Source: CAD feature listing. Evaluate the final solid. Frame: model axes, mm. Coordinates: 2 decimals unless noted, no trailing zeros. Loops run counter-clockwise (first coordinate to the right, second up) from the corner with the lowest first, then second, coordinate; pieces in that order, holes last. Notation, with made-up numbers: (41.5, 49) - (50.5, 49) arc R18 ccw to (50.5, 81) - close; hole circle Ø10 at (-8.75, 81). An arc over 180 degrees is marked (long way). Use CSV: the item, a comma, the result in double quotes. Start each with the question number.
```python
from build123d import *

# Parameters (mm, degrees)
F0_R     = 38.572234299
F1_DEPTH = 25.4
F2_DEPTH = 25.4
F3_DEPTH = 25.4


with BuildPart() as f1:
    # F0 (on Front) → F1 (new body)
    with BuildSketch(Plane.XZ):
        with Locations((-53.8619197905, 27.4006854743)):
            Circle(F0_R)
    extrude(amount=F1_DEPTH)

    # F2 (add): faces of the model
    f2_faces = [f1.faces().sort_by_distance(p)[0] for p in [
        (-53.8619197905, -25.4, 27.4006854743),
        (-53.8619197905, 0, 27.4006854743),
    ]]
    extrude(f2_faces, amount=F2_DEPTH, dir=(0, -1, 0))

    # F3 (add): a face of the model
    f3_faces = [f1.faces().sort_by_distance(p)[0] for p in [
        (-53.8619197905, 0, 27.4006854743),
    ]]
    extrude(f3_faces, amount=F3_DEPTH)


solid = f1.part
```
(1) Pin query (flat end, axial travel): pin 1 Ø3 at (y, z) = (-14.5, 33.5) entering from +X; pin 2 Ø1 at (x, y) = (-49.5, 8) entering from +Z; pin 3 Ø4 at (x, y) = (-38.5, -1) entering from -Z. Return the tip coordinate at first contact, or that it passes through.
(2) Section A-A on x = -22. Output: boundary loops of the cut face in (y, z), plus the area to 3 significant figures.
(3) Ray query, line 1 (Z direction, x = -53.5, y = 18); line 2 (Z direction, x = -34, y = -12.5); line 3 (X direction, y = -10, z = -2). Return the intervals inside material, ascending. Write a range as [from, to].
(4) Section B-B on z = 55.5. Output: boundary loops of the cut face in (x, y).
(5) Section C-C on y = -27. Output: boundary loops of the cut face in (x, z).
Solution:
1,pin 1,"stops at x = -15.56"
1,pin 2,"stops at z = 65.78"
1,pin 3,"stops at z = -8.78"
2,outline,"(-50.8, 5.66) - (25.4, 5.66) - (25.4, 49.14) - (-50.8, 49.14) - close"
2,area,"3,310 mm²"
3,line 1,"z = [-11.17, 65.97]"
3,line 2,"z = [-5.66, 60.47]"
3,line 3,"x = [-78.83, -28.89]"
4,outline,"(-80.29, -50.8) - (-27.44, -50.8) - (-27.44, 25.4) - (-80.29, 25.4) - close"
5,outline,"circle Ø77.14 at (-53.86, 27.4)"
